Verification items for this drawing (mm, ordinates from the low corner). A direction names the side the tool comes from. Round coordinates to 2 decimals unless told otherwise and drop trailing zeros. Loops run counter-clockwise (first coordinate to the right, second up) from the corner with the lowest first, then second, coordinate; pieces in that order, holes last. Notation, with made-up numbers: M 20,-37 L 74,-37 A32 ccw 74,-1 Z; hole C -18,82.5 d4. An arc over 180 degrees is marked long. Write item = value, one per line.
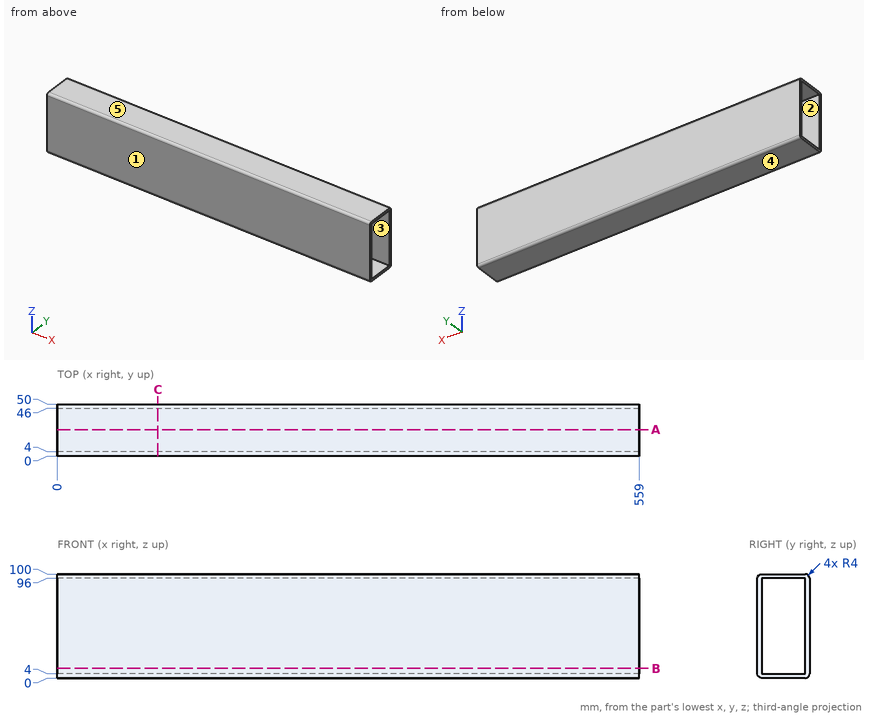
(1) Sectioned sample at B-B on z = 9.5. Record the cut outline in (x, y), then the cut area to 3 significant figures.
Result set:
outline = M 0,0 L 559,0 L 559,4 L 0,4 Z; M 0,46 L 559,46 L 559,50 L 0,50 Z
area = 4,470 mm2
(2) Depth check by flat-ended pin: pin 1 Ø12 at (y, z) = (28, 15) entering from -X. Enter the tip coordinate at first touch or a pass-through.
Result set:
pin_1 = through
(3) Material ranges on line 1 along Z through (x, y) = (59, 40.5); line 2 along Y through (x, z) = (429, 71.5), recorded low to high. Write a range as from..to.
Result set:
line_1 = 0..4, 96..100
line_2 = 0..4, 46..50
(4) Sectioned sample at A-A on y = 25.5. Record the cut outline in (x, z), then the cut area to 3 significant figures.
Result set:
outline = M 0,0 L 559,0 L 559,4 L 0,4 Z; M 0,96 L 559,96 L 559,100 L 0,100 Z
area = 4,470 mm2
(5) Release check for a two-part mould opening along Z. For the marked faces 3, 4 and 5 record: released by +Z, released by -Z, zero draft, split by the parting line, or undercut.
Result set:
face_3 = undercut
face_4 = released by -Z
face_5 = released by +Z
(6) Tool access check on the marked faces 1 and 2. Record the directions out of +Z, -Z, +X, -X, +Y, -Y that give a thin tool (end or side, any length) a straight path to the whole face; none if there is none.
Result set:
face_1 = +Z, -Z, +X, -X, -Y
face_2 = +X, -X
(7) Sectioned sample at C-C on x = 96.5. Record the cut outline in (y, z), then the cut area to 3 significant figures.
Result set:
outline = M 0,4 A4 ccw 4,0 L 46,0 A4 ccw 50,4 L 50,96 A4 ccw 46,100 L 4,100 A4 ccw 0,96 Z; hole M 4,4 L 46,4 L 46,96 L 4,96 Z
area = 1,120 mm2
